Source: CAD feature listing. Evaluate the final solid. Frame: model axes, mm. A direction names the side the tool comes from. Give positions to 0.01 mm unless a question says otherwise; leave off trailing zeros. Order: outer loops, then holes, each group sorted by start corner. A loop starts at its lowest first (then second) coordinate and runs counter-clockwise, first axis right, second up. Notation, with made-up numbers: (37, 14) -> (91, 14) arc R30 ccw to (91, 47) -> close; hole circle Ø5 at (-35, 46). An arc over 180 degrees is marked (long way). Answer in a Markdown table with one row per item.
Autodesk Inventor part; units mm, degrees
ref_plane "YZ Plane" through (0, 0, 0) normal (1, 0, 0) x (0, 1, 0)
ref_plane "XZ Plane" through (0, 0, 0) normal (0, 1, 0) x (-1, 0, 0)
ref_plane "XY Plane" through (0, 0, 0) normal (0, 0, 1) x (1, 0, 0)
sketch "Sketch1" plane through (0, 0, 0) normal (0, 1, 0) x (-1, 0, 0)
  line L0 (0, -5.4993) -> (-4.7625, -2.7496)
  line L1 (-4.7625, -2.7496) -> (-4.7625, 2.7496)
  line L2 (-4.7625, 2.7496) -> (0, 5.4993)
  line L3 (0, 5.4993) -> (4.7625, 2.7496)
  line L4 (4.7625, 2.7496) -> (4.7625, -2.7496)
  line L5 (4.7625, -2.7496) -> (0, -5.4993)
  circle A0 centre (0, 0) radius 2.0955
  dimension "d0" = 9.525
  dimension "d9" = 4.191
extrude "Extrusion1" add sketch "Sketch1" along normal blind 76.2
sketch "Sketch2" plane through (0, 76.2, 0) normal (0, 1, 0) x (1, 0, 0)
  circle A0 centre (0, 0) radius 3.175
  line L0 (-4.7625, 2.7496) -> (-4.7625, -2.7496)
  line L1 (-4.7625, -2.7496) -> (0, -5.4993)
  line L2 (0, -5.4993) -> (4.7625, -2.7496)
  line L3 (4.7625, -2.7496) -> (4.7625, 2.7496)
  line L4 (4.7625, 2.7496) -> (0, 5.4993)
  line L5 (0, 5.4993) -> (-4.7625, 2.7496)
  dimension "d3" = 6.35
extrude "Extrusion2" cut sketch "Sketch2" against normal blind 6.35
sketch "Sketch3" plane through (0, 0, 0) normal (0, -1, 0) x (1, 0, 0)
  circle A0 centre (0, 0) radius 3.175
  line L0 (-4.7625, -2.7496) -> (-4.7625, 2.7496)
  line L1 (0, -5.4993) -> (-4.7625, -2.7496)
  line L2 (4.7625, -2.7496) -> (0, -5.4993)
  line L3 (4.7625, 2.7496) -> (4.7625, -2.7496)
  line L4 (0, 5.4993) -> (4.7625, 2.7496)
  line L5 (-4.7625, 2.7496) -> (0, 5.4993)
  dimension "d6" = 6.35
extrude "Extrusion3" cut sketch "Sketch3" against normal blind 6.35
properties part number "PlanetShaft" material "Aluminum 6061"
(1) Section query A-A (y = 41.5). Return the cut outline in (x, z).
A:
| item | result |
|---|---|
| outline | (-4.76, -2.75) -> (0, -5.5) -> (4.76, -2.75) -> (4.76, 2.75) -> (0, 5.5) -> (-4.76, 2.75) -> close; hole circle Ø4.19 at (0, 0) |
(2) Pull-direction query (Z, two-part tool) for faces 1 (the cylindrical face through (-0.69, 73.07, 3.1)), 2 (the cylindrical face through (-2, 37.57, -0.63)), 3 (the flat face through (2.348, 37.656, -4.144)), 4 (the flat face through (0.8, 76.2, -2.1)); classes: +Z half, -Z half, draft (parallel to the pull), parting line (faces both ways), or undercut.
A:
| item | result |
|---|---|
| face 1 | parting line |
| face 2 | undercut |
| face 3 | -Z half |
| face 4 | draft |
(3) Access query for faces 5 (the flat face through (-4.762, 38, 0)), 6 (the flat face through (-3.2, 69.85, 1.1)), 7 (the cylindrical face through (-0.69, 3.13, -3.1)). Directions: +Z, -Z, +X, -X, +Y, -Y. A direction counts if a zero-diameter tool reaches every point of the face in a straight line with its end or side. Return the directions, or none.
A:
| item | result |
|---|---|
| face 5 | +Z, -Z, -X, +Y, -Y |
| face 6 | +Y |
| face 7 | -Y |
(4) First-contact query: pin 1 Ø2.5 at (x, z) = (0, 0) entering from -Y; pin 2 Ø1 at (x, y) = (-2.5, 43.5) entering from -Z; pin 3 Ø1.5 at (x, y) = (1.5, 50) entering from -Z. Flat tips, straight axial feed; report the tip coordinate or a pass-through.
A:
| item | result |
|---|---|
| pin 1 | passes through |
| pin 2 | stops at z = -4.34 |
| pin 3 | stops at z = -5.07 |
(5) Ray query, probe 1 along Z at (x, y) = (0, 60.5); probe 2 along Y at (x, z) = (0.5, 4); probe 3 along X at (y, z) = (67, -0.5). Return the intervals inside material, ascending.
A:
| item | result |
|---|---|
| probe 1 | z = -5.5 to -2.1, 2.1 to 5.5 |
| probe 2 | y = 6.35 to 69.85 |
| probe 3 | x = -4.76 to -2.03, 2.03 to 4.76 |
